from build123d import *

# Parameters (mm, degrees)
F0_R     = 7.5
F1_DEPTH = 8
F3_DEPTH = 100
F4_R     = 0.67804
F5_DEPTH = 100


with BuildPart() as f1:
    # F0 (on Top) → F1 (new body)
    with BuildSketch(Plane.XY):
        Circle(F0_R)
    extrude(amount=F1_DEPTH)

    # F2 (on face) → F3 (cut)
    with BuildSketch(Plane.XY.offset(8)):
        with BuildLine():
            ThreePointArc((0, 1.5), (0.274417, 1.474685), (0.539571, 1.399594))
            Line((0.539571, 1.399594), (2.231121, 5.027136))
            ThreePointArc((2.231121, 5.027136), (1.14034, 5.380485), (0, 5.5))
            Line((0, 5.5), (0, 1.5))
        make_face()
        with BuildLine():
            ThreePointArc((-1.299038, 0.75), (-1.139906, 0.974994), (-0.942299, 1.167079))
            Line((-0.942299, 1.167079), (-3.238067, 4.445776))
            ThreePointArc((-3.238067, 4.445776), (-4.089467, 3.677806), (-4.76314, 2.75))
            Line((-4.76314, 2.75), (-1.299038, 0.75))
        make_face()
        with BuildLine():
            Line((-4.76314, -2.75), (-1.299038, -0.75))
            ThreePointArc((-1.299038, -0.75), (-1.414323, -0.499691), (-1.481869, -0.232515))
            Line((-1.481869, -0.232515), (-5.469188, -0.58136))
            ThreePointArc((-5.469188, -0.58136), (-5.229807, -1.702679), (-4.76314, -2.75))
        make_face()
        with BuildLine():
            Line((0, -5.5), (0, -1.5))
            ThreePointArc((0, -1.5), (-0.274417, -1.474685), (-0.539571, -1.399594))
            Line((-0.539571, -1.399594), (-2.231121, -5.027136))
            ThreePointArc((-2.231121, -5.027136), (-1.14034, -5.380485), (0, -5.5))
        make_face()
        with BuildLine():
            Line((4.76314, -2.75), (1.299038, -0.75))
            ThreePointArc((1.299038, -0.75), (1.139906, -0.974994), (0.942299, -1.167079))
            Line((0.942299, -1.167079), (3.238067, -4.445776))
            ThreePointArc((3.238067, -4.445776), (4.089467, -3.677806), (4.76314, -2.75))
        make_face()
        with BuildLine():
            ThreePointArc((1.299038, 0.75), (1.414323, 0.499691), (1.481869, 0.232515))
            Line((1.481869, 0.232515), (5.469188, 0.58136))
            ThreePointArc((5.469188, 0.58136), (5.229807, 1.702679), (4.76314, 2.75))
            Line((4.76314, 2.75), (1.299038, 0.75))
        make_face()
    extrude(amount=-F3_DEPTH, mode=Mode.SUBTRACT)

    # F4 (on face) → F5 (cut)
    with BuildSketch(Plane.XY.offset(8)):
        Circle(F4_R)
    extrude(amount=-F5_DEPTH, mode=Mode.SUBTRACT)


solid = f1.part
For this review, take the finished solid that the model builds, in its own axes (mm). A direction names the side the tool comes from. Round coordinates to 2 decimals unless told otherwise and drop trailing zeros. Write each loop counter-clockwise with the first axis right and the second up, starting at its lowest first coordinate (ties: lowest second). Pieces come first, ordered by that corner, then holes. Notation, with made-up numbers: (10, 7.5) - (53, 7.5) arc R6 cw to (53, 18.5) - close; hole circle Ø3 at (63, 30.5). An arc over 180 degrees is marked (long way). Use a Markdown table: item, result.
Q1. Wall thickness on line 1 along Y through (x, z) = (-2.75, 7); line 2 along Y through (x, z) = (2.5, 7.75); line 3 along X through (y, z) = (-4, 0.5): over which ranges is each line inside the solid? List them lowest first.
Derived:
| item | result |
|---|---|
| line 1 | y = -6.98 to -1.59, -0.34 to 1.59, 3.75 to 6.98 |
| line 2 | y = -7.07 to -3.39, -1.44 to 0.32, 1.44 to 7.07 |
| line 3 | x = -6.34 to -1.75, 0 to 2.93, 3.77 to 6.34 |
Q2. Clearance check with flat-ended pins moving along their axes: pin 1 (1.5 mm diameter, centred on x = -0.5, z = 6.5, fed in from +Y); pin 2 (2 mm diameter, centred on y = -1.5, z = 3.5, fed in from +X); pin 3 (1.2 mm diameter, centred on y = -3.5, z = 2.5, fed in from -X); pin 4 (1.2 mm diameter, centred on y = 4.5, z = 3, fed in from +X). State where each tip first meets the part, or that it passes through.
Derived:
| item | result |
|---|---|
| pin 1 | stops at y = 7.5 |
| pin 2 | stops at x = 7.48 |
| pin 3 | stops at x = -6.92 |
| pin 4 | stops at x = 6.41 |
Q3. The part is to be moulded in two halves that separate along Y. For faces 3 (the cylindrical face through (-1.156, -5.377, 4.056)), 4 (the cylindrical face through (-7.493, 0.33, 3.944)), 5 (the flat face through (2, 0, 0)), say which applies: pulls with the +Y half, pulls with the -Y half, needs draft (parallel to the pull), parting line crosses it, or undercut.
Derived:
| item | result |
|---|---|
| face 3 | undercut |
| face 4 | parting line crosses it |
| face 5 | needs draft |
Q4. We need section D-D (x = 2.5). Give the boundary of the cut face in (y, z).
Derived:
| item | result |
|---|---|
| outline | (-7.07, 0) - (-3.39, 0) - (-3.39, 8) - (-7.07, 8) - close; (-1.44, 0) - (0.32, 0) - (0.32, 8) - (-1.44, 8) - close; (1.44, 0) - (7.07, 0) - (7.07, 8) - (1.44, 8) - close |
Q5. Machinability: for faces 1 (the flat face through (2, 0, 8)), 2 (the flat face through (3.4, 0.4, 4.1)), which of the approach directions +Z, -Z, +X, -X, +Y, -Y give a long, thin tool a straight path to every point of the face, cutting with its end or side? Answer none if there is none.
Derived:
| item | result |
|---|---|
| face 1 | +Z, +X, -X, +Y, -Y |
| face 2 | +Z, -Z |
Q6. We need section C-C (z = 3.25). Give the boundary of the cut face in (x, y).
Derived:
| item | result |
|---|---|
| outline | circle Ø15 at (0, 0); hole (-5.47, -0.58) arc R5.5 ccw to (-4.76, -2.75) - (-1.3, -0.75) arc R1.5 cw to (-1.48, -0.23) - close; hole (-4.76, 2.75) - (-1.3, 0.75) arc R1.5 cw to (-0.94, 1.17) - (-3.24, 4.45) arc R5.5 ccw to start; hole (-2.23, -5.03) arc R5.5 ccw to (0, -5.5) - (0, -1.5) arc R1.5 cw to (-0.54, -1.4) - close; hole circle Ø1.36 at (0, 0); hole (0, 1.5) arc R1.5 cw to (0.54, 1.4) - (2.23, 5.03) arc R5.5 ccw to (0, 5.5) - close; hole (0.94, -1.17) - (3.24, -4.45) arc R5.5 ccw to (4.76, -2.75) - (1.3, -0.75) arc R1.5 cw to start; hole (1.3, 0.75) arc R1.5 cw to (1.48, 0.23) - (5.47, 0.58) arc R5.5 ccw to (4.76, 2.75) - close |
Q7. We need section A-A (y = 0). Give the boundary of the cut face in (x, z).
Derived:
| item | result |
|---|---|
| outline | (-7.5, 0) - (-0.68, 0) - (-0.68, 8) - (-7.5, 8) - close; (0.68, 0) - (7.5, 0) - (7.5, 8) - (0.68, 8) - close |
Q8. We need section B-B (x = -1.75). Give the boundary of the cut face in (y, z).
Derived:
| item | result |
|---|---|
| outline | (-7.29, 0) - (-5.21, 0) - (-5.21, 8) - (-7.29, 8) - close; (-4, 0) - (-1.01, 0) - (-1.01, 8) - (-4, 8) - close; (-0.26, 0) - (1.01, 0) - (1.01, 8) - (-0.26, 8) - close; (2.32, 0) - (7.29, 0) - (7.29, 8) - (2.32, 8) - close |
